```python
from build123d import *

# Parameters (mm, degrees)
F0_W     = 16
F0_H     = 16
F1_DEPTH = 12.17
F2_W     = 9.64
F2_H     = 11.25
F3_DEPTH = 3.4


with BuildPart() as f1:
    # F0 (on Top) → F1 (new body)
    with BuildSketch(Plane.XY):
        Rectangle(F0_W, F0_H)
    extrude(amount=F1_DEPTH)

    # F2 (on face) → F3 (join)
    with BuildSketch(Plane.YZ.offset(8)):
        with Locations((0.12, 5.625)):
            Rectangle(F2_W, F2_H)
    extrude(amount=F3_DEPTH)


solid = f1.part
```
Geometry: final body of the model. Coordinates: model frame, mm. A direction names the side the tool comes from. Give positions to 0.01 mm unless a question says otherwise; leave off trailing zeros. Order: outer loops, then holes, each group sorted by start corner. A loop starts at its lowest first (then second) coordinate and runs counter-clockwise, first axis right, second up. Notation, with made-up numbers: M -7,47.25 L 12,47.25 A30 ccw 12,86.25 Z; hole C 46.25,61 d3. An arc over 180 degrees is marked long. Answer as CSV lines item,"result". Start each with the question number.
1) Cut plane B-B (y = -6.5). Output: boundary loops of the cut face in (x, z).
2) Set-up query: faces 1 (the flat face through (10, 0, 11.25)), 2 (the flat face through (10, -4.7, 6)), 3 (the flat face through (10, 4.94, 6)). Return all of +Z, -Z, +X, -X, +Y, -Y with unobstructed straight access to the full face (end or side cutting, diameter ignored); none if empty.
3) First-contact query: P1, Ø2.5, axis at x = 10.5, y = -2.5, coming from the +Z side; P2, Ø2.5, axis at x = 10.5, z = 6.5, coming from the +Y side; P3, Ø1.7, axis at x = 9, z = 7, coming from the -Y side. Flat tips, straight axial feed; report the tip coordinate or a pass-through.
4) Cut plane A-A (z = 1). Output: boundary loops of the cut face in (x, y), then the cut area to 3 significant figures.
5) Line query: line 1 (X direction, y = 5, z = 2.5); line 2 (Z direction, x = 8.75, y = -1.5); line 3 (Y direction, x = 10, z = 3). Output: solid intervals per line, ascending. Write a range as from..to.
Findings below:
1,outline,"M -8,0 L 8,0 L 8,12.17 L -8,12.17 Z"
2,face 1,"+Z, +X, +Y, -Y"
2,face 2,"+Z, -Z, +X, -Y"
2,face 3,"+Z, -Z, +X, +Y"
3,P1,"stops at z = 11.25"
3,P2,"stops at y = 4.94"
3,P3,"stops at y = -4.7"
4,outline,"M -8,-8 L 8,-8 L 8,-4.7 L 11.4,-4.7 L 11.4,4.94 L 8,4.94 L 8,8 L -8,8 Z"
4,area,"289 mm²"
5,line 1,"x = -8..8"
5,line 2,"z = 0..11.25"
5,line 3,"y = -4.7..4.94"
